from build123d import *

# Parameters (mm, degrees)
SKETCH1_R               = 1.65
SKETCH1_W               = 9
SKETCH1_H               = 9
SKETCH1_R_2             = 1.6
SKETCH1_R_3             = 3
SKETCH1_R_4             = 7.6
SKETCH1_R_5             = 2.6
BOSS_EXTRUDE1_DEPTH     = 3.175
FILLET1_R               = 10
CUT_EXTRUDE1_DEPTH      = 1
CUT_EXTRUDE1_DEPTH_BACK = 4.175
SKETCH3_R               = 1.65
BOSS_EXTRUDE2_DEPTH     = 3.175
FILLET2_R               = 3


with BuildPart() as part:
    # Sketch1 → Boss-Extrude1 (new body)
    with BuildSketch(Plane(origin=(0, 0, 0), x_dir=(1, 0, 0), z_dir=(0, 1, 0))):
        with BuildLine():
            Line((-51.31658538, 125.897213638), (-82.713802404, 110.430644428))
            Line((-82.713802404, 110.430644428), (-22.785408926, -11.224310227))
            ThreePointArc((-22.785408926, -11.224310227), (0, -25.4), (22.785408926, -11.224310227))
            Line((22.785408926, -11.224310227), (82.713802404, 110.430644428))
            Line((82.713802404, 110.430644428), (51.31658538, 125.897213638))
            Line((51.31658538, 125.897213638), (34.864798721, 92.5))
            Line((34.864798721, 92.5), (-34.864798721, 92.5))
            Line((-34.864798721, 92.5), (-51.31658538, 125.897213638))
        make_face()
        Polygon((-28.707179242, 80), (28.707179242, 80), (13, 48.114343343), (-13, 48.114343343), align=None, mode=Mode.SUBTRACT)
        with Locations((-8, -8)):
            Circle(SKETCH1_R, mode=Mode.SUBTRACT)
        Rectangle(SKETCH1_W, SKETCH1_H, mode=Mode.SUBTRACT)
        with Locations((-8, 8)):
            Circle(SKETCH1_R, mode=Mode.SUBTRACT)
        with Locations((-3.1, 20.76053754)):
            Circle(SKETCH1_R_2, mode=Mode.SUBTRACT)
        with Locations((8, -8)):
            Circle(SKETCH1_R, mode=Mode.SUBTRACT)
        with Locations((8, 8)):
            Circle(SKETCH1_R, mode=Mode.SUBTRACT)
        with Locations((17.5, 29.51053754)):
            Circle(SKETCH1_R_3, mode=Mode.SUBTRACT)
        with Locations((-30, 66.453060464)):
            Circle(SKETCH1_R, mode=Mode.SUBTRACT)
        with Locations((-60, 103.923048454)):
            Circle(SKETCH1_R_4, mode=Mode.SUBTRACT)
        with Locations((30, 66.453060464)):
            Circle(SKETCH1_R, mode=Mode.SUBTRACT)
        with Locations((60, 103.923048454)):
            Circle(SKETCH1_R_4, mode=Mode.SUBTRACT)
        with Locations((0, 86.25)):
            Circle(SKETCH1_R_5, mode=Mode.SUBTRACT)
        with Locations((-3.1, 38.26053754)):
            Circle(SKETCH1_R_2, mode=Mode.SUBTRACT)
    extrude(amount=BOSS_EXTRUDE1_DEPTH)

    # Fillet1
    fillet1_edges = [part.edges().sort_by_distance(p)[0] for p in [
        (51.31658538, 1.5875, -125.897213638),
        (82.713802404, 1.5875, -110.430644428),
        (-82.713802404, 1.5875, -110.430644428),
        (-51.31658538, 1.5875, -125.897213638),
    ]]
    fillet(fillet1_edges, radius=FILLET1_R)

    # Sketch2 → Cut-Extrude1 (cut, two sides)
    with BuildSketch(Plane(origin=(0, 3.175, 0), x_dir=(1, 0, 0), z_dir=(0, 1, 0))) as cut_extrude1_sk:
        Polygon((-45.79480762, 58.114343343), (-29.073580398, 58.114343343), (-12.254779912, 23.972089701), (-20.615393523, 7), align=None)
        Polygon((-62.733510758, 92.5), (-48.694138346, 64), (-40.333524735, 80.972089701), (-46.012283536, 92.5), align=None)
        Polygon((29.073580398, 58.114343343), (45.79480762, 58.114343343), (34.218483, 34.614343343), (25.857869389, 51.586433044), align=None)
        Polygon((46.012283536, 92.5), (62.733510758, 92.5), (48.694138346, 64), (40.333524735, 80.972089701), align=None)
    extrude(amount=CUT_EXTRUDE1_DEPTH, mode=Mode.SUBTRACT)
    extrude(cut_extrude1_sk.sketch, amount=-CUT_EXTRUDE1_DEPTH_BACK, mode=Mode.SUBTRACT)

    # Sketch3 → Boss-Extrude2 (add)
    with BuildSketch(Plane(origin=(0, 0, 0), x_dir=(1, 0, 0), z_dir=(0, 1, 0))):
        with BuildLine():
            Line((-69.257852251, 117.059174089), (-77.922641378, 125.361067209))
            Line((-77.922641378, 125.361067209), (-88.300007778, 114.5300808))
            Line((-88.300007778, 114.5300808), (-81.545013782, 108.057997365))
            Line((-81.545013782, 108.057997365), (-78.29478263, 101.460010992))
            ThreePointArc((-78.29478263, 101.460010992), (-78.792063776, 109.097507652), (-73.743168968, 114.849664202))
            Line((-73.743168968, 114.849664202), (-69.257852251, 117.059174089))
        make_face()
        with Locations((-78.17782959, 120.758363767)):
            Circle(SKETCH3_R, mode=Mode.SUBTRACT)
        with Locations((-83.712425003, 114.981837682)):
            Circle(SKETCH3_R, mode=Mode.SUBTRACT)
    extrude(amount=BOSS_EXTRUDE2_DEPTH)

    # Fillet2
    fillet2_edges = [part.edges().sort_by_distance(p)[0] for p in [
        (-81.545013782, 1.5875, -108.057997365),
        (-88.300007778, 1.5875, -114.5300808),
        (-77.922641378, 1.5875, -125.361067209),
        (-69.257852251, 1.5875, -117.059174089),
    ]]
    fillet(fillet2_edges, radius=FILLET2_R)


solid = part.part
Geometry check sheet. Reference: the model listing, model coordinates, mm. A direction names the side the tool comes from. Round coordinates to 2 decimals unless told otherwise and drop trailing zeros. Order: outer loops, then holes, each group sorted by start corner. A loop starts at its lowest first (then second) coordinate and runs counter-clockwise, first axis right, second up. Notation, with made-up numbers: M -10,18 L 37,18 A14 ccw 37,24 Z; hole C 35.25,30.25 d6. An arc over 180 degrees is marked long. Answer in a Markdown table with one row per item. Add a question column.
Item 1: Sectioned sample at A-A, the plane z = -45. Enter the section's corners in (x, y) (3 decimals).
Item 2: Depth check by flat-ended pin: pin 1 Ø1.6 at (x, y) = (-55.5, 2) entering from +Z; pin 2 Ø1.6 at (x, y) = (0.5, 2) entering from -Z; pin 3 Ø1 at (y, z) = (2, -1) entering from +X; pin 4 Ø5 at (x, z) = (17.5, -29.51) entering from -Y. Enter the tip coordinate at first touch or a pass-through.
Item 3: Set-up check for faces 5 (the face through (20.964, 1.565, -64.28)), 6 (the face through (67.109, 1.565, -118.118)): record each of +Z, -Z, +X, -X, +Y, -Y from which the full face is reachable in a straight line by a thin tool's end or side.
Item 4: Material ranges on L1, parallel to Z at x = 0, y = 1.75; L2, parallel to Z at x = 60, y = 1.45; L3, parallel to Z at x = -30, y = 1.1, recorded low to high. Write a range as [from, to].
Item 5: Draft check along Z on faces 1 (the face through (-40.797, 1.565, -104.542)), 2 (the face through (-5, 0, -34)), 3 (the face through (-44.57, 1.61, -72.37)), 4 (the face through (78.83, 1.61, -108.99)). Enter one of: released by +Z, released by -Z, zero draft, split by the parting line, or undercut.
Item 6: Sectioned sample at B-B, the plane x = 16.5. Enter the section's corners in (y, z) (3 decimals).
Item 7: Sectioned sample at C-C, the plane y = 1.9. State how many separate pieces and enclosed holes the cut face has, plus the area to 3 significant figures.
Filled in:
| question | item | result |
|---|---|---|
| 1 | outline | M -50.482,0 L -39.335,0 L -39.335,3.175 L -50.482,3.175 Z; M -22.613,0 L 29.102,0 L 29.102,3.175 L -22.613,3.175 Z; M 39.335,0 L 50.482,0 L 50.482,3.175 L 39.335,3.175 Z |
| 2 | pin 1 | stops at z = -53.56 |
| 2 | pin 2 | stops at z = -92.5 |
| 2 | pin 3 | stops at x = 29.05 |
| 2 | pin 4 | passes through |
| 3 | face 5 | +Y, -Y |
| 3 | face 6 | -Z, +X, +Y, -Y |
| 4 | L1 | z = [-92.5, -88.85], [-83.65, -80], [-48.11, -4.5], [4.5, 25.4] |
| 4 | L2 | z = [-121.61, -111.52], [-96.32, -92.5], [-86.95, -64.32] |
| 4 | L3 | z = [-92.5, -68.1], [-64.8, -58.11], [-26.05, -3.42] |
| 5 | face 1 | released by -Z |
| 5 | face 2 | zero draft |
| 5 | face 3 | undercut |
| 5 | face 4 | split by the parting line |
| 6 | outline | M 0,-92.5 L 3.175,-92.5 L 3.175,-80 L 0,-80 Z; M 0,-55.219 L 3.175,-55.219 L 3.175,-32.339 L 0,-32.339 Z; M 0,-26.682 L 3.175,-26.682 L 3.175,19.311 L 0,19.311 Z |
| 7 | separate pieces | 1 |
| 7 | enclosed holes | 20 |
| 7 | area | 9,020 mm² |
